from build123d import *

# Parameters (mm, degrees)
SKETCH1_W           = 20
SKETCH1_H           = 20
BOSS_EXTRUDE1_DEPTH = 20
SKETCH2_W           = 10
SKETCH2_H           = 10
CUT_EXTRUDE1_DEPTH  = 20
CUT_EXTRUDE2_DEPTH  = 20


with BuildPart() as part:
    # Sketch1 → Boss-Extrude1 (new body)
    with BuildSketch(Plane.XY):
        with Locations((10, 10)):
            Rectangle(SKETCH1_W, SKETCH1_H)
    extrude(amount=BOSS_EXTRUDE1_DEPTH)

    # Sketch2 → Cut-Extrude1 (cut)
    with BuildSketch(Plane(origin=(0, 20, 0), x_dir=(1, 0, 0), z_dir=(0, 1, 0))):
        with Locations((15, -15)):
            Rectangle(SKETCH2_W, SKETCH2_H)
    extrude(amount=-CUT_EXTRUDE1_DEPTH, mode=Mode.SUBTRACT)

    # Sketch3 → Cut-Extrude2 (cut)
    with BuildSketch(Plane(origin=(0, 20, 0), x_dir=(1, 0, 0), z_dir=(0, 1, 0))):
        Polygon((0, 0), (10, 0), (0, -5), align=None)
    extrude(amount=-CUT_EXTRUDE2_DEPTH, mode=Mode.SUBTRACT)


solid = part.part
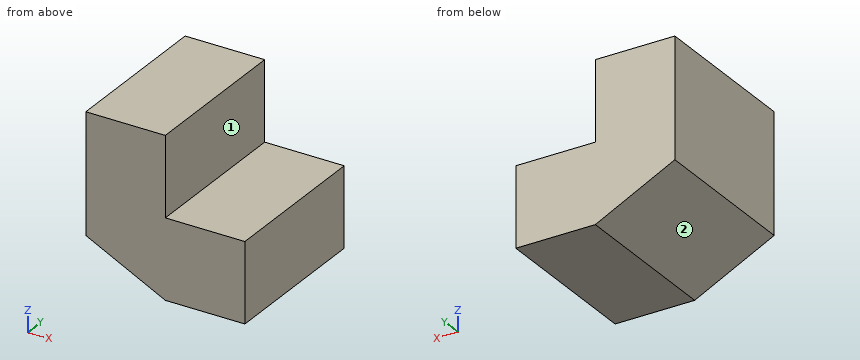
Can you work these out from the model? Positions are in its coordinate system, mm. Face numbers are marked on the shaded views. A direction names the side the tool comes from. Give positions to 0.01 mm unless a question says otherwise; leave off trailing zeros. Write each loop counter-clockwise with the first axis right and the second up, starting at its lowest first coordinate (ties: lowest second). Pieces come first, ordered by that corner, then holes. Notation, with made-up numbers: M 38.25,21 L 84.25,21 A4 ccw 84.25,28 Z; hole C -10,34.25 d10. An arc over 180 degrees is marked long. Answer in a Markdown table with one row per item. Add a question column.
Item 1: Imagine slicing it at C-C, the plane z = 2.5. Write out the boundary of the cut face in (x, y).
Item 2: Imagine slicing it at A-A, the plane y = 16. Write out the boundary of the cut face in (x, z), plus the area to 3 significant figures.
Item 3: Please list where these lines run through material, in increasing order: L1, parallel to Z at x = 17.75, y = 19; L2, parallel to Z at x = 8.75, y = 14.5 (3 decimals).
Item 4: For pin 1 Ø2 at (x, y) = (18, 9) entering from +Z; pin 2 Ø11 at (y, z) = (10, 16.5) entering from +X, each with a flat end and sliding along its axis, tell me the tip position at first contact or that it passes through.
Item 5: On a 3-axis mill with a long thin cutter (end or side, diameter ignored), from which of +Z, -Z, +X, -X, +Y, -Y can I reach the whole of each face in a straight line? I mean the marked faces 1 and 2. Say none if no direction works.
Item 6: Imagine slicing it at B-B, the plane x = 4. Write out the boundary of the cut face in (y, z), plus the area to 3 significant figures.
Evaluation:
| question | item | result |
|---|---|---|
| 1 | outline | M 5,0 L 20,0 L 20,20 L 5,20 Z |
| 2 | outline | M 0,5 L 10,0 L 20,0 L 20,10 L 10,10 L 10,20 L 0,20 Z |
| 2 | area | 275 mm² |
| 3 | L1 | z = 0 to 10 |
| 3 | L2 | z = 0.625 to 20 |
| 4 | pin 1 | stops at z = 10 |
| 4 | pin 2 | stops at x = 10 |
| 5 | face 1 | +Z, +X, +Y, -Y |
| 5 | face 2 | -Z, -X, +Y, -Y |
| 6 | outline | M 0,3 L 20,3 L 20,20 L 0,20 Z |
| 6 | area | 340 mm² |
